from build123d import *

# Parameters (mm, degrees)
SKETCH1_R                            = 75.692
SKETCH1_R_2                          = 69.342
BOSS_EXTRUDE1_DEPTH                  = 22.225
SKETCH2_R                            = 75.692
BOSS_EXTRUDE2_DEPTH                  = 12.7
TAP_DRILL_FOR_1_4_20_TAP1_AT_2_COUNT = 2
TAP_DRILL_FOR_1_4_20_TAP1_AT_2_PITCH = 53.488399339
CIRPATTERN1_COUNT                    = 6
F_1_2_0_5_DIAMETER_HOLE1_D           = 12.7
CUT_EXTRUDE1_DEPTH                   = 13.7000001


with BuildPart() as part:
    # Sketch1 → Boss-Extrude1 (new body)
    with BuildSketch(Plane(origin=(0, 0, 0), x_dir=(1, 0, 0), z_dir=(0, 1, 0))):
        Circle(SKETCH1_R)
        Circle(SKETCH1_R_2, mode=Mode.SUBTRACT)
    extrude(amount=BOSS_EXTRUDE1_DEPTH)

    # Sketch2 → Boss-Extrude2 (add)
    with BuildSketch(Plane.XZ):
        Circle(SKETCH2_R)
    extrude(amount=BOSS_EXTRUDE2_DEPTH)

    # Sketch4 → Tap Drill for 1/4-20 Tap1 (revolve, cut)
    with BuildSketch(Plane(origin=(73.997176623, 4.896298223, 15.927859738), x_dir=(0.210429897, 0, -0.97760895), z_dir=(0, 1, 0))):
        Polygon((0, 0), (0, 11.185816902), (2.5527, 9.652), (2.5527, 0), align=None)
    tap_drill_for_1_4_20_tap1 = revolve(axis=Axis((80.204993454, 4.896298223, 17.264089582), (-0.97760895, 0, -0.210429897)), mode=Mode.SUBTRACT)

    # Tap Drill for 1/4-20 Tap1 at 2: Tap Drill for 1/4-20 Tap1 ×2
    with Locations(*[Vector(-0.110438581, 0.851210999, 0.51307227) * (i * TAP_DRILL_FOR_1_4_20_TAP1_AT_2_PITCH) for i in range(1, TAP_DRILL_FOR_1_4_20_TAP1_AT_2_COUNT)]):
        add(tap_drill_for_1_4_20_tap1, mode=Mode.SUBTRACT)

    # CirPattern1: Tap Drill for 1/4-20 Tap1 ×6 about axis
    cirpattern1_axis = Axis((0, 22.225, 0), (0, -1, 0))
    for i in range(1, CIRPATTERN1_COUNT):
        add(tap_drill_for_1_4_20_tap1.rotate(cirpattern1_axis, i * 360 / CIRPATTERN1_COUNT), mode=Mode.SUBTRACT)

    # CirPattern1 copy 1 sketch → CirPattern1 copy 1 (revolve, cut)
    with BuildSketch(Plane(origin=(-3.515628412, 50.426212075, 80.653301416), x_dir=(0.951849134, 0, -0.306566839), z_dir=(0, 1, 0))):
        Polygon((0, 0), (0, 11.185816902), (2.5527, 9.652), (2.5527, 0), align=None)
    revolve(axis=Axis((-1.568928987, 50.426212075, 86.697543415), (-0.306566839, 0, -0.951849134)), mode=Mode.SUBTRACT)

    # CirPattern1 copy 2 sketch → CirPattern1 copy 2 (revolve, cut)
    with BuildSketch(Plane(origin=(-71.605622131, 50.426212075, 37.282027193), x_dir=(0.741419237, 0, 0.671042111), z_dir=(0, 1, 0))):
        Polygon((0, 0), (0, 11.185816902), (2.5527, 9.652), (2.5527, 0), align=None)
    revolve(axis=Axis((-75.866739537, 50.426212075, 41.990039348), (0.671042111, 0, -0.741419237)), mode=Mode.SUBTRACT)

    # CirPattern1 copy 3 sketch → CirPattern1 copy 3 (revolve, cut)
    with BuildSketch(Plane(origin=(-68.089993719, 50.426212075, -43.371274223), x_dir=(-0.210429897, 0, 0.97760895), z_dir=(0, 1, 0))):
        Polygon((0, 0), (0, 11.185816902), (2.5527, 9.652), (2.5527, 0), align=None)
    revolve(axis=Axis((-74.29781055, 50.426212075, -44.707504067), (0.97760895, 0, 0.210429897)), mode=Mode.SUBTRACT)

    # CirPattern1 copy 4 sketch → CirPattern1 copy 4 (revolve, cut)
    with BuildSketch(Plane(origin=(3.515628412, 50.426212075, -80.653301416), x_dir=(-0.951849134, 0, 0.306566839), z_dir=(0, 1, 0))):
        Polygon((0, 0), (0, 11.185816902), (2.5527, 9.652), (2.5527, 0), align=None)
    revolve(axis=Axis((1.568928987, 50.426212075, -86.697543415), (0.306566839, 0, 0.951849134)), mode=Mode.SUBTRACT)

    # CirPattern1 copy 5 sketch → CirPattern1 copy 5 (revolve, cut)
    with BuildSketch(Plane(origin=(71.605622131, 50.426212075, -37.282027193), x_dir=(-0.741419237, 0, -0.671042111), z_dir=(0, 1, 0))):
        Polygon((0, 0), (0, 11.185816902), (2.5527, 9.652), (2.5527, 0), align=None)
    revolve(axis=Axis((75.866739537, 50.426212075, -41.990039348), (-0.671042111, 0, 0.741419237)), mode=Mode.SUBTRACT)

    # 1/2 (0.5) Diameter Hole1 (through all)
    with Locations(Plane(origin=(0, 0, 0), x_dir=(1, 0, 0), z_dir=(0, 1, 0))):
        with Locations((0, -50.8)):
            Hole(F_1_2_0_5_DIAMETER_HOLE1_D / 2)

    # Sketch11 → Cut-Extrude1 (cut, through all)
    with BuildSketch(Plane(origin=(0, 0, 0), x_dir=(1, 0, 0), z_dir=(0, 1, 0))):
        with BuildLine():
            Line((-51.165057741, -3.071167846), (-42.54303006, 26.163931584))
            ThreePointArc((-42.54303006, 26.163931584), (-37.810889171, 28.740565552), (-35.234255202, 24.008424663))
            Line((-35.234255202, 24.008424663), (-43.856282883, -5.226674766))
            ThreePointArc((-43.856282883, -5.226674766), (-48.588423772, -7.803308735), (-51.165057741, -3.071167846))
        make_face()
        with BuildLine():
            Line((35.234255202, -24.008424663), (43.856282883, 5.226674766))
            ThreePointArc((43.856282883, 5.226674766), (48.588423772, 7.803308735), (51.165057741, 3.071167846))
            Line((51.165057741, 3.071167846), (42.54303006, -26.163931584))
            ThreePointArc((42.54303006, -26.163931584), (37.810889171, -28.740565552), (35.234255202, -24.008424663))
        make_face()
    extrude(amount=-CUT_EXTRUDE1_DEPTH, mode=Mode.SUBTRACT)


solid = part.part
Work out the finished part from the listing and answer in its coordinate system (mm). A direction names the side the tool comes from. Coordinates: 2 decimals unless noted, no trailing zeros. Write each loop counter-clockwise with the first axis right and the second up, starting at its lowest first coordinate (ties: lowest second). Pieces come first, ordered by that corner, then holes. Notation, with made-up numbers: M -30,40.5 L 28,40.5 A15 ccw 28,46.5 Z; hole C -14,14.5 d8. An arc over 180 degrees is marked long. Write item = value, one per line.
1. Determine the mould class of faces 4 (the face through (48.508, -6.261, -7.826)), 5 (the face through (-46.928, 5.874, 55.364)), 6 (the face through (33.3, 22.225, 61.3)) for opening direction Y: released by +Y, released by -Y, zero draft, split by the parting line, or undercut.
Solution:
face_4 = zero draft
face_5 = undercut
face_6 = released by +Y
2. The part is cut by section A-A (x = 0). Determine the outline of the cut face in (y, z) (3 decimals).
Solution:
outline = M -12.7,-75.692 L 22.225,-75.692 L 22.225,-69.342 L 0,-69.342 L 0,44.45 L -12.7,44.45 Z; M -12.7,57.15 L 0,57.15 L 0,69.342 L 22.225,69.342 L 22.225,75.692 L -12.7,75.692 Z
3. For faces 1 (the face through (-20.45, 3.17, -69.62)), 2 (the face through (-1, 0, 1)), 3 (the face through (39.485, -6.261, 9.596)), determine the directions among +Z, -Z, +X, -X, +Y, -Y from which every point of the face is accessible in a straight line to the end or side of a thin tool.
Solution:
face_1 = none
face_2 = +Y
face_3 = +Y, -Y
4. The part is cut by section C-C (z = 0). Determine the outline of the cut face in (x, y) (3 decimals).
Solution:
outline = M -75.692,-12.7 L -50.259,-12.7 L -50.259,0 L -69.342,0 L -69.342,22.225 L -75.692,22.225 Z; M -42.315,-12.7 L 42.315,-12.7 L 42.315,0 L -42.315,0 Z; M 50.259,-12.7 L 75.692,-12.7 L 75.692,22.225 L 69.342,22.225 L 69.342,0 L 50.259,0 Z
5. The part is cut by section D-D (z = 40.5). Determine the outline of the cut face in (x, y) (3 decimals).
Solution:
outline = M -63.946,-12.7 L 63.946,-12.7 L 63.946,22.225 L 56.286,22.225 L 56.286,0 L -56.286,0 L -56.286,22.225 L -63.946,22.225 Z
6. Straight lines are drawn through the part: line 1 (X direction, y = 13.5, z = 0); line 2 (Z direction, x = 41, y = 0.5); line 3 (Z direction, x = 15, y = 6). For each, find the intervals that lie inside material, in ascending order. Write a range as from..to.
Solution:
line_1 = -75.69..-69.34, 69.34..75.69
line_2 = -63.63..-55.92, 55.92..63.63
line_3 = -74.19..-67.7, 67.7..74.19
7. The part is cut by section B-B (y = -4). Determine the outline of the cut face in (x, z), then the cut area to 3 significant figures.
Solution:
outline = C 0,0 d151.38; hole M -51.17,3.07 L -42.54,-26.16 A3.81 ccw -35.23,-24.01 L -43.86,5.23 A3.81 ccw Z; hole C 0,50.8 d12.7; hole M 35.23,24.01 L 43.86,-5.23 A3.81 ccw 51.17,-3.07 L 42.54,26.16 A3.81 ccw Z
area = 17,300 mm2
8. Flat-ended cylindrical pins translate along their axes: pin 1 (4 mm diameter, centred on x = 35.5, z = 29.5, fed in from +Y); pin 2 (4 mm diameter, centred on y = 3, z = -21.5, fed in from +X); pin 3 (10 mm diameter, centred on x = 46, y = 18, fed in from +Z); pin 4 (7.5 mm diameter, centred on x = 0, z = 50.8, fed in from -Y). Find the tip coordinate at first contact, or state that the pin passes through.
Solution:
pin_1 = 0
pin_2 = 73.14
pin_3 = 63.63
pin_4 = through
